from build123d import *

# Parameters (mm, degrees)
ESQUISSE1_W             = 45
ESQUISSE1_H             = 45
BOSS_EXTRU_1_DEPTH      = 10
ESQUISSE2_W             = 39
ESQUISSE2_H             = 39
ENL_V_MAT_EXTRU_1_DEPTH = 65.420493634
PER_AGE1_D              = 4.9175
PER_AGE2_D              = 4.9175
PER_AGE2_DEPTH          = 45
PER_AGE3_D              = 4.9175
CHANFREIN1_SIZE         = 0.54125
ESQUISSE9_W             = 19.5
ESQUISSE9_H             = 10
ENL_V_MAT_EXTRU_2_DEPTH = 10
ESQUISSE10_W            = 10
ESQUISSE10_H            = 19.5
ENL_V_MAT_EXTRU_3_DEPTH = 10


with BuildPart() as part:
    # Esquisse1 → Boss.-Extru.1 (new body)
    with BuildSketch(Plane(origin=(0, 0, -5), x_dir=(-1, 0, 0), z_dir=(0, 0, -1))):
        with Locations((-22.5, 22.5)):
            Rectangle(ESQUISSE1_W, ESQUISSE1_H)
    extrude(amount=-BOSS_EXTRU_1_DEPTH)

    # Esquisse2 → Enlèv. mat.-Extru.1 (cut, through all)
    with BuildSketch(Plane.XY.offset(5)):
        with Locations((25.5, 25.5)):
            Rectangle(ESQUISSE2_W, ESQUISSE2_H)
    extrude(amount=-ENL_V_MAT_EXTRU_1_DEPTH, mode=Mode.SUBTRACT)

    # Perçage1 (through all)
    with Locations(Plane(origin=(0, 6, 0), x_dir=(1, 0, 0), z_dir=(0, 1, 0))):
        with Locations((35, 0), (15, 0)):
            Hole(PER_AGE1_D / 2)

    # Perçage2
    with Locations(Plane.ZY):
        with Locations((0, 15)):
            Hole(PER_AGE2_D / 2, depth=PER_AGE2_DEPTH)

    # Perçage3 (through all)
    with Locations(Plane(origin=(6, 0, 0), x_dir=(0, 0, -1), z_dir=(1, 0, 0))):
        with Locations((0, 35)):
            Hole(PER_AGE3_D / 2)

    # Chanfrein1
    chanfrein1_edges = [part.edges().sort_by_distance(p)[0] for p in [
        (17.45875, 6, 0),
        (17.45875, 0, 0),
        (37.45875, 6, 0),
        (37.45875, 0, 0),
        (6, 15, 2.45875),
        (0, 15, 2.45875),
        (6, 35, -2.45875),
        (0, 35, -2.45875),
    ]]
    chamfer(chanfrein1_edges, length=CHANFREIN1_SIZE)

    # Esquisse9 → Enlèv. mat.-Extru.2 (cut)
    with BuildSketch(Plane(origin=(0, 6, 0), x_dir=(1, 0, 0), z_dir=(0, 1, 0))):
        with Locations((35.25, 0)):
            Rectangle(ESQUISSE9_W, ESQUISSE9_H)
    extrude(amount=-ENL_V_MAT_EXTRU_2_DEPTH, mode=Mode.SUBTRACT)

    # Esquisse10 → Enlèv. mat.-Extru.3 (cut)
    with BuildSketch(Plane(origin=(6, 0, 0), x_dir=(0, 0, -1), z_dir=(1, 0, 0))):
        with Locations((0, 35.25)):
            Rectangle(ESQUISSE10_W, ESQUISSE10_H)
    extrude(amount=-ENL_V_MAT_EXTRU_3_DEPTH, mode=Mode.SUBTRACT)


solid = part.part
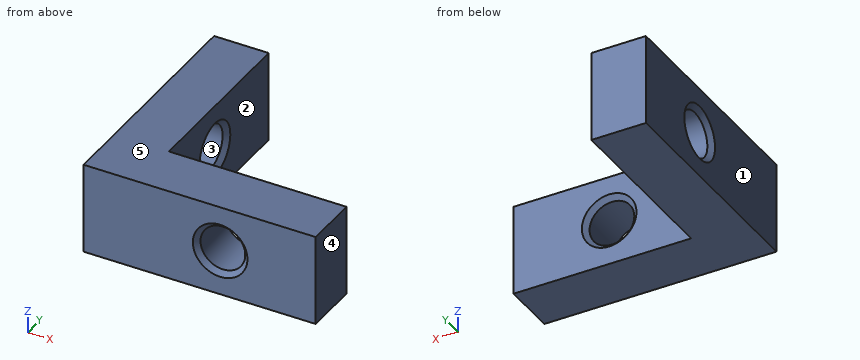
Input: part model. Units: mm. Frame: model coordinates. Face numbers are marked on the shaded views. A direction names the side the tool comes from. Give positions to 0.01 mm unless a question says otherwise; leave off trailing zeros. Loops run counter-clockwise (first coordinate to the right, second up) from the corner with the lowest first, then second, coordinate; pieces in that order, holes last. Notation, with made-up numbers: M 0,14 L 23,14 A22 ccw 23,36 Z; hole C -39,56 d3. An arc over 180 degrees is marked long. Use one line per item in the form item = value.
1. Section query D-D, the plane x = 3.5. Return the cut outline in (y, z).
Numbers:
outline = M 0,-5 L 25.5,-5 L 25.5,5 L 0,5 Z; hole C 15,0 d4.92
2. Pull-direction query (Z, two-part tool) for the marked faces 3, 4 and 5; classes: released by +Z, released by -Z, zero draft, split by the parting line, or undercut.
Numbers:
face_3 = undercut
face_4 = zero draft
face_5 = released by +Z
3. Line query: L1, parallel to X at y = 4.25, z = 0; L2, parallel to Z at x = 15, y = 3.4. Output: solid intervals per line, ascending.
Numbers:
L1 = 0 to 12.54, 17.46 to 25.5
L2 = -5 to -2.46, 2.46 to 5
4. First-contact query: pin 1 (1.5 mm diameter, centred on x = 8.5, z = 2, fed in from +Y); pin 2 (5.5 mm diameter, centred on y = 15, z = 0, fed in from +X). Flat tips, straight axial feed; report the tip coordinate or a pass-through.
Numbers:
pin_1 = 6
pin_2 = 5.75
5. Section query A-A, the plane x = 15. Return the cut outline in (y, z).
Numbers:
outline = M 0,-5 L 6,-5 L 6,-3 L 5.46,-2.46 L 0.54,-2.46 L 0,-3 Z; M 0,3 L 0.54,2.46 L 5.46,2.46 L 6,3 L 6,5 L 0,5 Z
6. Reachability of the marked faces 1 and 2 from +Z, -Z, +X, -X, +Y, -Y: full face, straight path, thin tool, end or side. Return the list, or none.
Numbers:
face_1 = +Z, -Z, -X, +Y, -Y
face_2 = +Z, -Z, +X, +Y
7. Section query C-C, the plane z = 0. Return the cut outline in (x, y).
Numbers:
outline = M 0,0 L 12,0 L 12.54,0.54 L 12.54,5.46 L 12,6 L 6,6 L 6,12 L 5.46,12.54 L 0.54,12.54 L 0,12 Z; M 0,18 L 0.54,17.46 L 5.46,17.46 L 6,18 L 6,25.5 L 0,25.5 Z; M 17.46,0.54 L 18,0 L 25.5,0 L 25.5,6 L 18,6 L 17.46,5.46 Z
